from build123d import *

# Parameters (mm, degrees)
F0_R     = 63
F0_R_2   = 60
F1_DEPTH = 2
F2_DEPTH = 12
F5_DEPTH = 10


with BuildPart() as f1:
    # F0 (on Top) → F1 (new body)
    with BuildSketch(Plane.XY):
        with BuildLine():
            Line((65, 65), (-65, 65))
            Line((-65, 65), (-65, -65))
            Line((-65, -65), (65, -65))
            Line((65, -65), (65, -15.0111682118))
            ThreePointArc((65, -15.0111682118), (63.0170909154, -12.5652293358), (65, -10.1192904598))
            Line((65, -10.1192904598), (65, 65))
        make_face()
        Circle(F0_R, mode=Mode.SUBTRACT)
        Circle(F0_R)
        Circle(F0_R_2, mode=Mode.SUBTRACT)
    extrude(amount=F1_DEPTH)

    # F0 (on Top) → F2 (join)
    with BuildSketch(Plane.XY):
        Circle(F0_R)
        Circle(F0_R_2, mode=Mode.SUBTRACT)
    extrude(amount=F2_DEPTH)

    # F3 (on Right) → F4 (revolve)
    with BuildSketch(Plane.YZ):
        Polygon((47, 72), (60, 12), (63, 12), (50, 72), align=None)
    revolve(axis=Axis((0, 0, 42), (0, 0, 1)))

    # F5 (add): a face of the model
    f5_faces = [f1.faces().sort_by_distance(p)[0] for p in [
        (0, -48.5857864376, 72),
    ]]
    extrude(f5_faces, amount=F5_DEPTH)


solid = f1.part
Input: part model. Units: mm. Frame: model coordinates. A direction names the side the tool comes from. Give positions to 0.01 mm unless a question says otherwise; leave off trailing zeros. Loops run counter-clockwise (first coordinate to the right, second up) from the corner with the lowest first, then second, coordinate; pieces in that order, holes last. Notation, with made-up numbers: (35.25, 9) - (65.25, 9) arc R20 cw to (65.25, 46) - close; hole circle Ø11 at (-33, 3). An arc over 180 degrees is marked (long way). Use CSV: the item, a comma, the result in double quotes. Start each with the question number.
Item 1: Section D-D on z = 40.5. Return loops of the section in (x, y) (3 decimals), then the cut area to 3 significant figures.
Item 2: Section C-C on z = 74.5. Return loops of the section in (x, y).
Item 3: Line query: line 1 (Y direction, x = 0, z = 7.25); line 2 (X direction, y = 0, z = 77). Output: solid intervals per line, ascending.
Item 4: Contact query for flat-ended pins moving along their axis: P1, Ø5, axis at x = -36, z = 64, coming from the +Y side; P2, Ø10, axis at y = -51, z = 20.5, coming from the +X side; P3, Ø12, axis at x = -22.5, z = 13, coming from the -Y side. Output: stop coordinate, or through.
Item 5: Section A-A on y = 0. Return loops of the section in (x, z), then the cut area to 3 significant figures.
Item 6: Reachability of faces 1 (the cylindrical face through (-59.94, 2.64, 5.92)), 2 (the cylindrical face through (-15.02, 47.69, 76.93)), 3 (the flat face through (33, -34, 82)) from +Z, -Z, +X, -X, +Y, -Y: full face, straight path, thin tool, end or side. Return the list, or none.
Item 7: Mould query, pull axis Y, two halves, no side actions, for faces 4 (the cylindrical face through (-8.201, 62.464, 6.93)), 5 (the cylindrical face through (-14.12, 44.83, 76.93)), 6 (the conical face through (44.98, 23.4, 54.91)), 7 (the flat face through (-63, -5, 2)). Classes: pulls with the +Y half, pulls with the -Y half, needs draft (parallel to the pull), parting line crosses it, or undercut.
Ans:
1,outline,"circle Ø113.65 at (0, 0); hole circle Ø107.65 at (0, 0)"
1,area,"1,040 mm2"
2,outline,"circle Ø100 at (0, 0); hole circle Ø94 at (0, 0)"
3,line 1,"y = -63 to -60, 60 to 63"
3,line 2,"x = -50 to -47, 47 to 50"
4,P1,"stops at y = 39.54"
4,P2,"stops at x = 40.54"
4,P3,"stops at y = -60.78"
5,outline,"(-65, 0) - (-60, 0) - (-60, 12) - (-47, 72) - (-47, 82) - (-50, 82) - (-50, 72) - (-63, 12) - (-63, 2) - (-65, 2) - close; (47, 72) - (60, 12) - (60, 0) - (65, 0) - (65, 2) - (63, 2) - (63, 12) - (50, 72) - (50, 82) - (47, 82) - close"
5,area,"500 mm2"
6,face 1,"-Z"
6,face 2,"+Z"
6,face 3,"+Z, +X, -X, +Y, -Y"
7,face 4,"parting line crosses it"
7,face 5,"undercut"
7,face 6,"undercut"
7,face 7,"needs draft"
